from build123d import *

# Parameters (mm, degrees)
CROQUIS1_W              = 16
CROQUIS1_H              = 40
CROQUIS1_R              = 2.55
SALIENTE_EXTRUIR1_DEPTH = 1.8
CROQUIS2_W              = 16
CROQUIS2_H              = 1.8
SALIENTE_EXTRUIR2_DEPTH = 38.2
CROQUIS3_R              = 2.55
CORTAR_EXTRUIR1_DEPTH   = 38.2
REDONDEO1_R             = 1
REDONDEO2_R             = 9
REDONDEO3_R             = 1


with BuildPart() as part:
    # Croquis1 → Saliente-Extruir1 (new body)
    with BuildSketch(Plane(origin=(0, 0, 0), x_dir=(0, 0, -1), z_dir=(1, 0, 0))):
        with Locations((-8, 20)):
            Rectangle(CROQUIS1_W, CROQUIS1_H)
        with Locations((-8, 31.5)):
            Circle(CROQUIS1_R, mode=Mode.SUBTRACT)
        with Locations((-8, 13.5)):
            Circle(CROQUIS1_R, mode=Mode.SUBTRACT)
    extrude(amount=SALIENTE_EXTRUIR1_DEPTH)

    # Croquis2 → Saliente-Extruir2 (add)
    with BuildSketch(Plane(origin=(1.8, 0, 0), x_dir=(0, 0, -1), z_dir=(1, 0, 0))):
        with Locations((-8, 0.9)):
            Rectangle(CROQUIS2_W, CROQUIS2_H)
    extrude(amount=SALIENTE_EXTRUIR2_DEPTH)

    # Croquis3 → Cortar-Extruir1 (cut)
    with BuildSketch(Plane(origin=(0, 1.8, 0), x_dir=(1, 0, 0), z_dir=(0, 1, 0))):
        with Locations(Location((31.5, -8, 0), (0, 0, 270))):
            Circle(CROQUIS3_R)
        with Locations(Location((13.5, -8, 0), (0, 0, 270))):
            Circle(CROQUIS3_R)
    extrude(amount=-CORTAR_EXTRUIR1_DEPTH, mode=Mode.SUBTRACT)

    # Redondeo1
    redondeo1_edges = [part.edges().sort_by_distance(p)[0] for p in [
        (1.8, 1.8, 8),
    ]]
    fillet(redondeo1_edges, radius=REDONDEO1_R)

    # Redondeo2
    # the kernel refuses this fillet: 9 mm, written as the material it takes off along each edge
    with BuildSketch(Plane(origin=(40, 24.3, 16), x_dir=(0, 0, -1), z_dir=(0, -1, 0)), Plane(origin=(-22.5, 40, 0), x_dir=(0, -1, 0), z_dir=(1, 0, 0)), Plane(origin=(-22.5, 40, 16), x_dir=(0, 0, -1), z_dir=(1, 0, 0))) as redondeo2_piece_1:
        with BuildLine():
            CenterArc((REDONDEO2_R, -REDONDEO2_R), REDONDEO2_R, 90, 90)
            Line((0, -REDONDEO2_R), (0, 0))
            Line((0, 0), (REDONDEO2_R, 0))
        make_face()
    extrude(amount=46.8, mode=Mode.SUBTRACT)
    with BuildSketch(Plane(origin=(40, -22.5, 0), x_dir=(-1, 0, 0), z_dir=(0, 1, 0))) as redondeo2_piece_2:
        with BuildLine():
            CenterArc((REDONDEO2_R, REDONDEO2_R), REDONDEO2_R, 180, 90)
            Line((0, REDONDEO2_R), (0, 0))
            Line((0, 0), (REDONDEO2_R, 0))
        make_face()
    extrude(amount=46.8, mode=Mode.SUBTRACT)

    # Redondeo3
    redondeo3_edges = [part.edges().sort_by_distance(p)[0] for p in [
        (0, 0, 8),
    ]]
    fillet(redondeo3_edges, radius=REDONDEO3_R)


solid = part.part
For this review, take the finished solid that the model builds, in its own axes (mm). A direction names the side the tool comes from. Round coordinates to 2 decimals unless told otherwise and drop trailing zeros. Loops run counter-clockwise (first coordinate to the right, second up) from the corner with the lowest first, then second, coordinate; pieces in that order, holes last. Notation, with made-up numbers: (11, 24) - (37, 24) arc R26 cw to (37, 54) - close; hole circle Ø1 at (4.25, 24.5). An arc over 180 degrees is marked (long way). Use one line per item in the form item = value.
1) Tool access review of faces 1 (the face through (0.301, 0.285, 7.888)), 2 (the face through (21, 1.8, 8)): name each direction out of +Z, -Z, +X, -X, +Y, -Y from which nothing blocks a thin tool from reaching the whole face with its end or side.
Solutions:
face_1 = +Z, -Z, -X, -Y
face_2 = +Z, -Z, +X, +Y
2) We need section D-D on z = 3. Write out the cut boundary in (x, y).
Solutions:
outline = (0, 1) arc R1 ccw to (1, 0) - (37.71, 0) - (37.71, 1.8) - (2.8, 1.8) arc R1 cw to (1.8, 2.8) - (1.8, 37.71) - (0, 37.71) - close
3) Mouldability with a two-part tool opening along Z and no side actions: class faces 3 (the face through (37.068, 0.913, 13.647)), 4 (the face through (0.89, 11.24, 6.82)), 5 (the face through (1.8, 22, 8)), 6 (the face through (34.03, 0.91, 7.67)) as pulls with the +Z half, pulls with the -Z half, needs draft (parallel to the pull), parting line crosses it, or undercut.
Solutions:
face_3 = pulls with the +Z half
face_4 = undercut
face_5 = needs draft
face_6 = undercut
4) We need section C-C on z = 6.5. Write out the cut boundary in (x, y), then the cut area to 3 significant figures.
Solutions:
outline = (0, 1) arc R1 ccw to (1, 0) - (11.44, 0) - (11.44, 1.8) - (2.8, 1.8) arc R1 cw to (1.8, 2.8) - (1.8, 11.44) - (0, 11.44) - close; (0, 15.56) - (1.8, 15.56) - (1.8, 29.44) - (0, 29.44) - close; (0, 33.56) - (1.8, 33.56) - (1.8, 39.65) - (0, 39.65) - close; (15.56, 0) - (29.44, 0) - (29.44, 1.8) - (15.56, 1.8) - close; (33.56, 0) - (39.65, 0) - (39.65, 1.8) - (33.56, 1.8) - close
area = 110 mm2
5) Clearance check with flat-ended pins moving along their axes: P1, Ø3, axis at y = 31.5, z = 8, coming from the +X side; P2, Ø2, axis at y = 24, z = 13, coming from the +X side; P3, Ø4, axis at x = 33, z = 14, coming from the +Y side. State where each tip first meets the part, or that it passes through.
Solutions:
P1 = through
P2 = 1.8
P3 = 1.8
6) We need section A-A on y = 13.5. Write out the cut boundary in (x, z), then the cut area to 3 significant figures.
Solutions:
outline = (0, 0) - (1.8, 0) - (1.8, 5.45) - (0, 5.45) - close; (0, 10.55) - (1.8, 10.55) - (1.8, 16) - (0, 16) - close
area = 19.6 mm2
7) Wall thickness on probe 1 along X at (y, z) = (0.8, 8); probe 2 along Y at (x, z) = (6, 1); probe 3 along Z at (x, y) = (1, 13): over which ranges is each line inside the solid? List them lowest first.
Solutions:
probe_1 = 0.02 to 10.95, 16.05 to 28.95, 34.05 to 39.94
probe_2 = 0 to 1.8
probe_3 = 0 to 5.5, 10.5 to 16
